Work out the finished part from the listing and answer in its coordinate system (mm). Coordinates: 2 decimals unless noted, no trailing zeros. Order: outer loops, then holes, each group sorted by start corner. A loop starts at its lowest first (then second) coordinate and runs counter-clockwise, first axis right, second up.
1. The part is cut by section B-B, the plane x = 35. Give the vertices of the cut face in (y, z).
2. A flat-ended cylindrical pin translates along its axis: pin 1 Ø0.5 at (x, y) = (51, -0.5) entering from +Z. Find the tip coordinate at first contact, or state that the pin passes through.
3. The part is cut by section A-A, the plane y = -2.4. Give the vertices of the cut face in (x, z).
4. Find the intervals of material crossed by probe 1 along Z at (x, y) = (-48, -1.45); probe 2 along Z at (x, y) = (46, -0.4); probe 3 along Y at (x, z) = (32, -1.35), in increasing order.
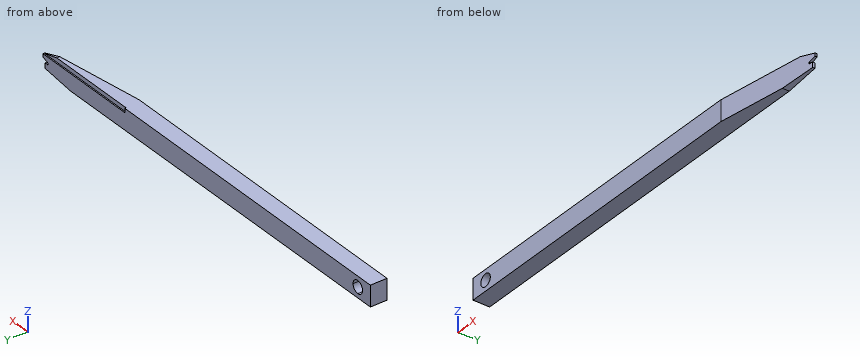
```python
from build123d import *

# Parameters (mm, degrees)
F0_W      = 104
F0_H      = 5
F1_DEPTH  = 4
F3_DEPTH  = 4
F4_W      = 0.65
F4_H      = 3.25
F5_DEPTH  = 4
F7_DEPTH  = 4
F8_W      = 1
F8_H      = 0.4
F9_DEPTH  = 4
F10_W     = 0.65
F10_H     = 0.6
F11_DEPTH = 4
F13_DEPTH = 4
F15_DEPTH = 4
F17_DEPTH = 5.001
F18_R     = 0.1
F20_DEPTH = 0.3


with BuildPart() as f1:
    # F0 (on Front) → F1 (new body)
    with BuildSketch(Plane.XZ):
        Rectangle(F0_W, F0_H)
    extrude(amount=F1_DEPTH)

    # F2 (on face) → F3 (cut, through all)
    with BuildSketch(Plane.XZ.offset(4)):
        with BuildLine():
            ThreePointArc((-48, -1.5), (-46.9393398282, -1.0606601718), (-46.5, 0))
            ThreePointArc((-46.5, 0), (-49.0606601718, 1.0606601718), (-48, -1.5))
        make_face()
    extrude(amount=-F3_DEPTH, mode=Mode.SUBTRACT)

    # F4 (on face) → F5 (cut, through all)
    with BuildSketch(Plane.XZ.offset(4)):
        with Locations((51.675, -0.875)):
            Rectangle(F4_W, F4_H)
    extrude(amount=-F5_DEPTH, mode=Mode.SUBTRACT)

    # F6 (on face) → F7 (cut, through all)
    with BuildSketch(Plane.XZ.offset(4)):
        Polygon((43.205653572, -2.5), (51.35, -2.5), (51.35, -1.5), align=None)
    extrude(amount=-F7_DEPTH, mode=Mode.SUBTRACT)

    # F8 (on face) → F9 (cut, through all)
    with BuildSketch(Plane.XZ.offset(4)):
        with Locations((50.85, -0.05)):
            Rectangle(F8_W, F8_H)
    extrude(amount=-F9_DEPTH, mode=Mode.SUBTRACT)

    # F10 (on face) → F11 (join)
    with BuildSketch(Plane.XZ.offset(4)):
        with Locations((51.675, 0.45)):
            Rectangle(F10_W, F10_H)
    extrude(amount=-F11_DEPTH)

    # F12 (on face) → F13 (cut, through all)
    with BuildSketch(Plane.XZ.offset(4)):
        Polygon((52, 0.15), (52, 0.75), (50.35, 0.15), align=None)
    extrude(amount=-F13_DEPTH, mode=Mode.SUBTRACT)

    # F14 (on face) → F15 (cut, through all)
    with BuildSketch(Plane.XZ.offset(4)):
        Polygon((52, 1.5), (52, 2.5), (48, 2.5), align=None)
    extrude(amount=-F15_DEPTH, mode=Mode.SUBTRACT)

    # F16 (on face) → F17 (cut, through all)
    with BuildSketch(Plane.XY.offset(2.5)):
        Polygon((52, -4), (52, -0.45), (26.7404374855, -4), align=None)
    extrude(amount=-F17_DEPTH, mode=Mode.SUBTRACT)

    # F18
    f18_edges = [f1.edges().sort_by_distance(p)[0] for p in [
        (50.35, -0.340946, -0.25),
    ]]
    fillet(f18_edges, radius=F18_R)

    # F19 (on face) → F20 (cut)
    with BuildSketch(Plane(origin=(0, 0, 0), x_dir=(-1, 0, 0), z_dir=(0, 1, 0))):
        Polygon((-48, 2.5), (-52, 1.5), (-26, 1.5), (-26, 2.5), align=None)
    extrude(amount=-F20_DEPTH, mode=Mode.SUBTRACT)


solid = f1.part
```
Geometry says:
1. outline: (-2.84, -2.5) - (0, -2.5) - (0, 1.5) - (-0.3, 1.5) - (-0.3, 2.5) - (-2.84, 2.5) - close
2. pin 1: stops at z = 1.81
3. outline: (-52, -2.5) - (38.13, -2.5) - (38.13, 2.5) - (-52, 2.5) - close; hole circle Ø3 at (-48, 0)
4. probe 1: z = -2.5 to -1.5, 1.5 to 2.5
4. probe 2: z = -2.16 to 2.5
4. probe 3: y = -3.26 to 0
